Part model, mm, in its own coordinate system. A direction names the side the tool comes from. Give positions to 0.01 mm unless a question says otherwise; leave off trailing zeros. Order: outer loops, then holes, each group sorted by start corner. A loop starts at its lowest first (then second) coordinate and runs counter-clockwise, first axis right, second up.
1. Slice it at A-A on z = 0. List the corners of the cut face in (x, y), and give its area (3 significant figures).
2. Slice it at D-D on y = 14.25. List the corners of the cut face in (x, z), and give its area (3 significant figures).
3. Drop flat-ended pins along their axis: pin 1 Ø1 at (x, y) = (-6, 10) entering from +Z; pin 2 Ø6 at (x, y) = (-15.5, 14) entering from +Z; pin 3 Ø12 at (y, z) = (5.5, 9.5) entering from +X. Give the stop position or say it passes through.
4. Slice it at B-B on x = -31. List the corners of the cut face in (y, z).
5. Mould opens along X. For faces 1 (the cylindrical face through (17.235, 3.042, 41.569)), 2 (the flat face through (-14, 0, -43)), 3 (the cylindrical face through (14.418, 11.832, 45.783)) say: +X half, -X half, draft (parallel to the pull), parting line (faces both ways), or undercut.
6. Which spindle directions (+Z, -Z, +X, -X, +Y, -Y) get a long thin tool onto all of the face, cutting with end or side? Do faces 4 (the flat face through (-14, 24, -43)), 5 (the cylindrical face through (-17.235, 21.535, 41.569)), 6 (the flat face through (40, 6, -14)). Say none if no direction does.
7. Probe line 1 (X direction, y = 20.3, z = 0); line 2 (X direction, y = 14.75, z = 0); line 3 (Z direction, x = -32, y = 19.75). List the from-to ranges inside material, lowest first.
8. Slice it at C-C on y = 3.5. List the corners of the cut face in (x, z).
from build123d import *

# Parameters (mm, degrees)
SKIZZE1_R                       = 48
SKIZZE1_R_2                     = 42
AUFSATZ_LINEAR_AUSTRAGEN2_DEPTH = 24
SKIZZE2_R                       = 45
SCHNITT_LINEAR_AUSTRAGEN1_DEPTH = 5
SCHNITT_LINEAR_START            = -6
SKIZZE4_R                       = 45
SCHNITT_LINEAR_AUSTRAGEN2_DEPTH = 6


with BuildPart() as part:
    # Skizze1 → Aufsatz-Linear austragen2 (new body)
    with BuildSketch(Plane(origin=(0, 0, 0), x_dir=(1, 0, 0), z_dir=(0, 1, 0))):
        with Locations(Location((0, 0, 0), (0, 0, 270))):
            Circle(SKIZZE1_R)
        with Locations(Location((0, 0, 0), (0, 0, 270))):
            Circle(SKIZZE1_R_2, mode=Mode.SUBTRACT)
    extrude(amount=AUFSATZ_LINEAR_AUSTRAGEN2_DEPTH)

    # Skizze2 → Schnitt-Linear austragen1 (cut)
    with BuildSketch(Plane(origin=(0, 24, 0), x_dir=(1, 0, 0), z_dir=(0, 1, 0))):
        with Locations(Location((0, 0, 0), (0, 0, 270))):
            Circle(SKIZZE2_R)
    extrude(amount=-SCHNITT_LINEAR_AUSTRAGEN1_DEPTH, mode=Mode.SUBTRACT)

    # Skizze4 → Schnitt-Linear austragen2 (cut)
    with BuildSketch(Plane.XZ.offset(SCHNITT_LINEAR_START)):
        with Locations(Location((0, 0, 0), (0, 0, 90))):
            Circle(SKIZZE4_R)
    extrude(amount=SCHNITT_LINEAR_AUSTRAGEN2_DEPTH, mode=Mode.SUBTRACT)


solid = part.part
Data:
1. outline: (-48, 0) - (-45, 0) - (-45, 6) - (-42, 6) - (-42, 19) - (-45, 19) - (-45, 24) - (-48, 24) - close; (42, 6) - (45, 6) - (45, 0) - (48, 0) - (48, 24) - (45, 24) - (45, 19) - (42, 19) - close
1. area: 222 mm2
2. outline: circle Ø96 at (0, 0); hole circle Ø84 at (0, 0)
2. area: 1,700 mm2
3. pin 1: stops at z = 47.68
3. pin 2: stops at z = 46.34
3. pin 3: stops at x = 47.87
4. outline: (0, -36.65) - (24, -36.65) - (24, -32.62) - (19, -32.62) - (19, -28.34) - (6, -28.34) - (6, -32.62) - (0, -32.62) - close; (0, 32.62) - (6, 32.62) - (6, 28.34) - (19, 28.34) - (19, 32.62) - (24, 32.62) - (24, 36.65) - (0, 36.65) - close
5. face 1: undercut
5. face 2: draft
5. face 3: parting line
6. face 4: +Z, -Z, +X, -X, +Y
6. face 5: +Y
6. face 6: -Y
7. line 1: x = -48 to -45, 45 to 48
7. line 2: x = -48 to -42, 42 to 48
7. line 3: z = -35.78 to -31.64, 31.64 to 35.78
8. outline: circle Ø96 at (0, 0); hole circle Ø90 at (0, 0)
